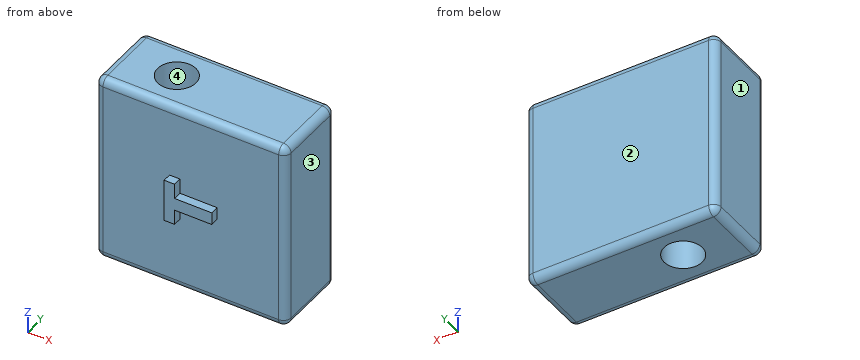
```python
from build123d import *

# Parameters (mm, degrees)
F0_W     = 127
F0_H     = 127
F1_DEPTH = 50.8
F2_R     = 5.08
F4_DEPTH = 5.66607
F6_DEPTH = 127.001


with BuildPart() as f1:
    # F0 (on Front) → F1 (new body)
    with BuildSketch(Plane.XZ):
        with Locations((0.4741810262, -5.6527711832)):
            Rectangle(F0_W, F0_H)
    extrude(amount=F1_DEPTH)

    # F2
    f2_edges = [f1.edges().sort_by_distance(p)[0] for p in [
        (0.474181, -50.8, -69.152771),
        (0.474181, 0, -69.152771),
        (0.474181, 0, 57.847229),
        (0.474181, -50.8, 57.847229),
        (-63.025819, -50.8, -5.652771),
        (-63.025819, 0, -5.652771),
        (-63.025819, -25.4, 57.847229),
        (-63.025819, -25.4, -69.152771),
        (63.974181, -25.4, -69.152771),
        (63.974181, -25.4, 57.847229),
        (63.974181, 0, -5.652771),
        (63.974181, -50.8, -5.652771),
    ]]
    fillet(f2_edges, radius=F2_R)

    # F3 (on face) → F4 (join)
    with BuildSketch(Plane.XZ.offset(50.8)):
        Polygon((-13.6571113464, 8.5772094634), (-13.6571113464, -19.8827518299), (-6.7716367987, -19.8827518299), (-6.7716367987, -9.7840579375), (18.0160704556, -9.7840579375), (18.0160704556, -1.521484429), (-6.7716367987, -1.521484429), (-6.7716367987, 8.5772094634), align=None)
    extrude(amount=F4_DEPTH)

    # F5 (on face) → F6 (cut, through all)
    with BuildSketch(Plane(origin=(0, 0, -69.1527711832), x_dir=(1, 0, 0), z_dir=(0, 0, -1))):
        with BuildLine():
            ThreePointArc((-37.6258189738, 25.4), (-24.9258189738, 12.7), (-12.2258189738, 25.4))
            ThreePointArc((-12.2258189738, 25.4), (-24.9258189738, 38.1), (-37.6258189738, 25.4))
        make_face()
    extrude(amount=-F6_DEPTH, mode=Mode.SUBTRACT)


solid = f1.part
```
Work out the finished part from the listing and answer in its coordinate system (mm). Face numbers are marked on the shaded views. Round coordinates to 2 decimals unless told otherwise and drop trailing zeros. Write each loop counter-clockwise with the first axis right and the second up, starting at its lowest first coordinate (ties: lowest second). Pieces come first, ordered by that corner, then holes. Notation, with made-up numbers: (20.25, 36.25) - (57.25, 36.25) arc R34 ccw to (57.25, 67.25) - close; hole circle Ø1 at (-1, 15). An arc over 180 degrees is marked (long way). Return JSON: item names as keys, results as strings. Group by question number.
Q1. The part is cut by section B-B on z = 41. Write down the section's boundary in (x, y).
Q2. The part is cut by section A-A on y = -25.4. Write down the section's boundary in (x, z), then the cut area to 3 significant figures.
Q3. The part is cut by section D-D on x = -32. Write down the section's boundary in (y, z).
Q4. The part is cut by section C-C on x = 14.5. Write down the section's boundary in (y, z).
Q5. Find the intervals of material crossed by L1, parallel to X at y = -25.4, z = 20; L2, parallel to Y at x = -3, z = 21; L3, parallel to X at y = -32, z = -24, in increasing order.
Q6. Each of these flat-tipped pins is pushed along its axis until it touches: pin 1 Ø6 at (x, y) = (2, -53) entering from +Z; pin 2 Ø3 at (x, y) = (-9, -54.5) entering from +Z; pin 3 Ø1.7 at (y, z) = (-54.5, -5.5) entering from -X; pin 4 Ø1.5 at (x, y) = (-27.5, -14) entering from -Z. Where does it stop, or does it pass through?
Q7. The mould has two halves that part along X. Classify the marked faces 1, 2, 3 and 4: released by +X, released by -X, zero draft, split by the parting line, or undercut.
Solved:
{
 "1": {"outline": "(-63.03, -45.72) arc R5.08 ccw to (-57.95, -50.8) - (58.89, -50.8) arc R5.08 ccw to (63.97, -45.72) - (63.97, -5.08) arc R5.08 ccw to (58.89, 0) - (-57.95, 0) arc R5.08 ccw to (-63.03, -5.08) - close; hole circle Ø25.4 at (-24.93, -25.4)"},
 "2": {"outline": "(-63.03, -64.07) arc R5.08 ccw to (-57.95, -69.15) - (-37.63, -69.15) - (-37.63, 57.85) - (-57.95, 57.85) arc R5.08 ccw to (-63.03, 52.77) - close; (-12.23, -69.15) - (58.89, -69.15) arc R5.08 ccw to (63.97, -64.07) - (63.97, 52.77) arc R5.08 ccw to (58.89, 57.85) - (-12.23, 57.85) - close", "area": "12,900 mm²"},
 "3": {"outline": "(-50.8, -64.07) arc R5.08 ccw to (-45.72, -69.15) - (-35.95, -69.15) - (-35.95, 57.85) - (-45.72, 57.85) arc R5.08 ccw to (-50.8, 52.77) - close; (-14.85, -69.15) - (-5.08, -69.15) arc R5.08 ccw to (0, -64.07) - (0, 52.77) arc R5.08 ccw to (-5.08, 57.85) - (-14.85, 57.85) - close"},
 "4": {"outline": "(-56.47, -9.78) - (-50.8, -9.78) - (-50.8, -64.07) arc R5.08 ccw to (-45.72, -69.15) - (-5.08, -69.15) arc R5.08 ccw to (0, -64.07) - (0, 52.77) arc R5.08 ccw to (-5.08, 57.85) - (-45.72, 57.85) arc R5.08 ccw to (-50.8, 52.77) - (-50.8, -1.52) - (-56.47, -1.52) - close"},
 "5": {"L1": "-63.03 to -37.63, -12.23 to 63.97", "L2": "-50.8 to 0", "L3": "-63.03 to -35.78, -14.08 to 63.97"},
 "6": {"pin 1": "z = 55.5", "pin 2": "z = 8.58", "pin 3": "x = -13.66", "pin 4": "through"},
 "7": {"face 1": "released by -X", "face 2": "zero draft", "face 3": "released by +X", "face 4": "undercut"}
}
